```python
from build123d import *

# Parameters (mm, degrees)
CUT_EXTRUDE1_START = -8
CUT_EXTRUDE1_DEPTH = 8


with BuildPart() as part:
    # Sketch2 → Revolve3 (revolve)
    with BuildSketch(Plane.XY):
        Polygon((-42.25, 12.4), (-15.4, 12.4), (-15.4, 12.1), (15.4, 12.1), (15.4, 0), (-54.7, 0), (-54.7, 2), (-44.8, 2), (-44.8, 3.475), (-42.25, 3.475), align=None)
    revolve(axis=Axis((-28.825, 0, 0), (-1, 0, 0)))

    # Sketch3 → Cut-Extrude1 (cut)
    with BuildSketch(Plane.ZY.offset(54.7).offset(CUT_EXTRUDE1_START)):
        with BuildLine():
            Line((-1.322875656, 1.5), (1.322875656, 1.5))
            ThreePointArc((1.322875656, 1.5), (0, 2), (-1.322875656, 1.5))
        make_face()
    extrude(amount=CUT_EXTRUDE1_DEPTH, mode=Mode.SUBTRACT)


solid = part.part
```
CAD build for the part. Positions are in the model's coordinates, mm. A direction names the side the tool comes from. Round coordinates to 2 decimals unless told otherwise and drop trailing zeros. Write each loop counter-clockwise with the first axis right and the second up, starting at its lowest first coordinate (ties: lowest second). Pieces come first, ordered by that corner, then holes. Notation, with made-up numbers: (39.25, -9) - (53.25, -9) arc R27 cw to (53.25, 30) - close; hole circle Ø3 at (51, -16.75). An arc over 180 degrees is marked (long way). Return JSON: item names as keys, results as strings. Group by question number.
Item 1: Band-saw the part on C-C on x = -18.5. List the corners of the cut face in (y, z), plus the area to 3 significant figures.
Item 2: Flat gauge pins, fed straight in: pin 1 Ø2 at (x, z) = (0, -7) entering from +Y; pin 2 Ø0.8 at (x, z) = (-51, 0.5) entering from +Y; pin 3 Ø7.5 at (y, z) = (6, 5.5) entering from -X. Where does each tip first touch, or does it go through?
Item 3: Band-saw the part on B-B on y = 0. List the corners of the cut face in (x, z) (3 decimals).
Item 4: Band-saw the part on D-D on z = -6. List the corners of the cut face in (x, y), plus the area to 3 significant figures.
Item 5: 3-axis set-ups, long thin cutter, end or side, ignore diameter. For faces 1 (the face through (0.22, 11.18, 4.63)), 2 (the face through (-42.25, -3, 3)), 3 (the face through (-51, 1.5, 0)): which of +Z, -Z, +X, -X, +Y, -Y reach the whole face in a straight line?
Item 6: Band-saw the part on A-A on z = 0. List the corners of the cut face in (x, y) (3 decimals), plus the area to 3 significant figures.
Item 7: Probe probe 1 along X at (y, z) = (2.25, 4); probe 2 along Z at (x, y) = (-42.5, 0) (3 decimals); probe 3 along X at (y, z) = (-1, -3). List the from-to ranges inside material, lowest first.
Resolved:
{
 "1": {"outline": "circle Ø24.8 at (0, 0)", "area": "483 mm²"},
 "2": {"pin 1": "stops at y = 10.51", "pin 2": "stops at y = 1.5", "pin 3": "stops at x = -42.25"},
 "3": {"outline": "(-54.7, -2) - (-44.8, -2) - (-44.8, -3.475) - (-42.25, -3.475) - (-42.25, -12.4) - (-15.4, -12.4) - (-15.4, -12.1) - (15.4, -12.1) - (15.4, 12.1) - (-15.4, 12.1) - (-15.4, 12.4) - (-42.25, 12.4) - (-42.25, 3.475) - (-44.8, 3.475) - (-44.8, 2) - (-54.7, 2) - close"},
 "4": {"outline": "(-42.25, -10.85) - (-15.4, -10.85) - (-15.4, -10.51) - (15.4, -10.51) - (15.4, 10.51) - (-15.4, 10.51) - (-15.4, 10.85) - (-42.25, 10.85) - close", "area": "1,230 mm²"},
 "5": {"face 1": "+X", "face 2": "-X", "face 3": "+Z, -Z, -X, +Y"},
 "6": {"outline": "(-54.7, -2) - (-44.8, -2) - (-44.8, -3.475) - (-42.25, -3.475) - (-42.25, -12.4) - (-15.4, -12.4) - (-15.4, -12.1) - (15.4, -12.1) - (15.4, 12.1) - (-15.4, 12.1) - (-15.4, 12.4) - (-42.25, 12.4) - (-42.25, 3.475) - (-44.8, 3.475) - (-44.8, 2) - (-46.7, 2) - (-46.7, 1.5) - (-54.7, 1.5) - close", "area": "1,460 mm²"},
 "7": {"probe 1": "x = -42.25 to 15.4", "probe 2": "z = -3.475 to 3.475", "probe 3": "x = -44.8 to 15.4"}
}
